Build history of the part. All positions in model axes, mm. Coordinates: 2 decimals unless noted, no trailing zeros. Loops run counter-clockwise (first coordinate to the right, second up) from the corner with the lowest first, then second, coordinate; pieces in that order, holes last. Notation, with made-up numbers: (32.25, 48.5) - (59.25, 48.5) arc R17 ccw to (59.25, 63.5) - close; hole circle Ø6 at (-25.75, 83.5). An arc over 180 degrees is marked (long way). One line per item, written item: value.
```python
from build123d import *

# Parameters (mm, degrees)
SM_BASE_FLANGE_1_DEPTH = 16


# Sheet-metal steps are written as plain solids
with BuildPart() as part:
    # Sketch 1 → 基体-法兰1 (new body)
    with BuildSketch(Plane(origin=(0, 0, 0), x_dir=(0, 0, -1), z_dir=(1, 0, 0))):
        Polygon((0, 0), (0, 280), (4, 280), (488, 20), (488, 0), align=None)
    extrude(amount=-SM_BASE_FLANGE_1_DEPTH)


solid = part.part
```
Item 1: Cut at C-C, the plane y = 53. Write the cut outline in (x, z).
Check result:
outline: (-16, -426.57) - (0, -426.57) - (0, 0) - (-16, 0) - close
Item 2: Probe probe 1 along Y at (x, z) = (-14.25, -154); probe 2 along Z at (x, y) = (-13.5, 257.5); probe 3 along Z at (x, y) = (-6, 28). List the from-to ranges inside material, lowest first. Write a range as from..to.
Check result:
probe 1: y = 0..199.42
probe 2: z = -45.88..0
probe 3: z = -473.11..0
Item 3: Drop flat-ended pins along their axis: P1, Ø3, axis at x = -6.5, y = 96, coming from the -Z side; P2, Ø4, axis at x = -4.5, z = -141.5, coming from the +Y side; P3, Ø8, axis at x = -12, z = -224.5, coming from the +Y side. Give the stop position or say it passes through.
Check result:
P1: stops at z = -349.32
P2: stops at y = 207.21
P3: stops at y = 163.7
Item 4: Cut at A-A, the plane x = -6.75. Write the cut outline in (y, z).
Check result:
outline: (0, -488) - (20, -488) - (280, -4) - (280, 0) - (0, 0) - close
Item 5: Cut at B-B, the plane z = -397. Write the cut outline in (x, y).
Check result:
outline: (-16, 0) - (0, 0) - (0, 68.88) - (-16, 68.88) - close
